```python
from build123d import *

# Parameters (mm, degrees)
BOSS_EXTRUDE1_DEPTH = 95
SKETCH3_W           = 10
SKETCH3_H           = 10
CUT_EXTRUDE2_DEPTH  = 3
SKETCH4_W           = 40
SKETCH4_H           = 25
SKETCH4_H_2         = 60
CUT_EXTRUDE8_DEPTH  = 2
SKETCH5_W           = 14
SKETCH5_H           = 50
CUT_EXTRUDE9_DEPTH  = 2
SKETCH6_R           = 0.825
CUT_EXTRUDE10_DEPTH = 203.435174809


with BuildPart() as part:
    # Sketch1 → Boss-Extrude1 (new body)
    with BuildSketch(Plane(origin=(0, 0, 0), x_dir=(1, 0, 0), z_dir=(0, 1, 0))):
        Polygon((0, 0), (0, 66), (14, 66), (14, 68), (-16, 68), (-16, 66), (-2, 66), (-2, 0), (-16, 0), (-16, -2), (14, -2), (14, 0), align=None)
    extrude(amount=BOSS_EXTRUDE1_DEPTH)

    # Sketch3 → Cut-Extrude2 (cut)
    with BuildSketch(Plane.XZ):
        with Locations((-1, 0)):
            Rectangle(SKETCH3_W, SKETCH3_H)
        with Locations((-1, -66)):
            Rectangle(SKETCH3_W, SKETCH3_H)
    extrude(amount=-CUT_EXTRUDE2_DEPTH, mode=Mode.SUBTRACT)

    # Mirror2: part across plane


with BuildPart() as part_1:
    add(part.part)
    add(part.part.mirror(Plane(origin=(0, 95, 0), x_dir=(0, 0, 1), z_dir=(0, -1, 0))))

    # Sketch4 → Cut-Extrude8 (cut)
    with BuildSketch(Plane.ZY.offset(2)):
        with Locations((-33, 154.5)):
            Rectangle(SKETCH4_W, SKETCH4_H)
        with Locations((-33, 63)):
            Rectangle(SKETCH4_W, SKETCH4_H_2)
    extrude(amount=-CUT_EXTRUDE8_DEPTH, mode=Mode.SUBTRACT)

    # Sketch5 → Cut-Extrude9 (cut)
    with BuildSketch(Plane(origin=(0, 0, 0), x_dir=(-1, 0, 0), z_dir=(0, 0, -1))):
        with Locations((-7, 165)):
            Rectangle(SKETCH5_W, SKETCH5_H)
    extrude(amount=-CUT_EXTRUDE9_DEPTH, mode=Mode.SUBTRACT)

    # Sketch6 → Cut-Extrude10 (cut, through all)
    with BuildSketch(Plane.ZY.offset(2)):
        with Locations((-25.5, 123.074804834)):
            Circle(SKETCH6_R)
        with Locations((-40.5, 123.074804834)):
            Circle(SKETCH6_R)
    extrude(amount=-CUT_EXTRUDE10_DEPTH, mode=Mode.SUBTRACT)


solid = part_1.part
```
Design review of the part built by this model. Coordinates are the model's own, in mm. A direction names the side the tool comes from. Round coordinates to 2 decimals unless told otherwise and drop trailing zeros. Order: outer loops, then holes, each group sorted by start corner. A loop starts at its lowest first (then second) coordinate and runs counter-clockwise, first axis right, second up. Notation, with made-up numbers: (40, 68.5) - (55, 68.5) arc R35 cw to (55, 100.5) - close; hole circle Ø5 at (8, 32). An arc over 180 degrees is marked (long way). One line per question, with ' | ' between items.
Item 1: For P1, Ø3, axis at x = -2.5, z = -2, coming from the +Y side; P2, Ø0.6, axis at x = -0.5, y = 188, coming from the +Z side; P3, Ø12, axis at y = 67.5, z = -8, coming from the +X side, all flat-tipped, find the tip position at first contact; note any pin that passes through.
Checks:
P1: y = 187 | P2: z = -5 | P3: x = 0
Item 2: Machinability: for faces 5 (the face through (7, 71, 0)), 6 (the face through (-1, 187, -66)), 7 (the face through (-9, 96, -66)), 8 (the face through (-1, 3, -66)), which of the approach directions +Z, -Z, +X, -X, +Y, -Y give a long, thin tool a straight path to every point of the face, cutting with its end or side? Answer none if there is none.
Checks:
face 5: +X, +Y, -Y | face 6: -Z, +Y | face 7: -X, +Y, -Y | face 8: -Z, -Y
Item 3: Take a section at A-A, the plane x = 11.25. Write out the cut boundary in (y, z), then the cut area to 3 significant figures.
Checks:
outline: (0, -68) - (190, -68) - (190, -66) - (0, -66) - close; (0, 0) - (140, 0) - (140, 2) - (0, 2) - close | area: 660 mm²
Item 4: Take a section at C-C, the plane z = -16. Write out the cut boundary in (x, y).
Checks:
outline: (-2, 0) - (0, 0) - (0, 33) - (-2, 33) - close; (-2, 93) - (0, 93) - (0, 142) - (-2, 142) - close; (-2, 167) - (0, 167) - (0, 190) - (-2, 190) - close
Item 5: Take a section at D-D, the plane x = -9. Write out the cut boundary in (y, z), then the cut area to 3 significant figures.
Checks:
outline: (0, -68) - (190, -68) - (190, -66) - (0, -66) - close; (0, 0) - (190, 0) - (190, 2) - (0, 2) - close | area: 760 mm²
Item 6: Wall thickness on line 1 (Z direction, x = -14.5, y = 38); line 2 (Y direction, x = -1.2, z = -40.5); line 3 (X direction, y = 140, z = -15): over which ranges is each line inside the solid? List them lowest first. Write a range as [from, to].
Checks:
line 1: [-68, -66], [0, 2] | line 2: [0, 33], [93, 122.25], [123.9, 142], [167, 190] | line 3: [-2, 0]
Item 7: Take a section at B-B, the plane y = 47. Write out the cut boundary in (x, z), then the cut area to 3 significant figures.
Checks:
outline: (-16, -68) - (14, -68) - (14, -66) - (0, -66) - (0, -53) - (-2, -53) - (-2, -66) - (-16, -66) - close; (-16, 0) - (-2, 0) - (-2, -13) - (0, -13) - (0, 0) - (14, 0) - (14, 2) - (-16, 2) - close | area: 172 mm²
Item 8: Draft analysis for pull direction Z (two halves, no side actions). For faces 1 (the face through (0, 96, -32)), 2 (the face through (-1.7, 187, -0.7)), 3 (the face through (-1, 96, 2)), 4 (the face through (-1, 96, -68)), state which applies: +Z half, -Z half, draft (parallel to the pull), parting line (faces both ways), or undercut.
Checks:
face 1: undercut | face 2: draft | face 3: +Z half | face 4: -Z half
